Input: dimensioned drawing with shaded views. Units: mm. Origin: part minimum x, y, z. Round coordinates to 2 decimals unless told otherwise and drop trailing zeros. Loops run counter-clockwise (first coordinate to the right, second up) from the corner with the lowest first, then second, coordinate; pieces in that order, holes last.
Item 1: Section query C-C on x = 56.5. Return loops of the section in (y, z).
Item 2: Ray query, L1, parallel to X at y = 77.5, z = 1.25; L2, parallel to Y at x = 53.5, z = 5.5. Return the intervals inside material, ascending.
Item 3: Section query A-A on z = 8.5. Return loops of the section in (x, y).
Item 4: Section query B-B on y = 68.5. Return loops of the section in (x, z), then the cut area to 3 significant figures.
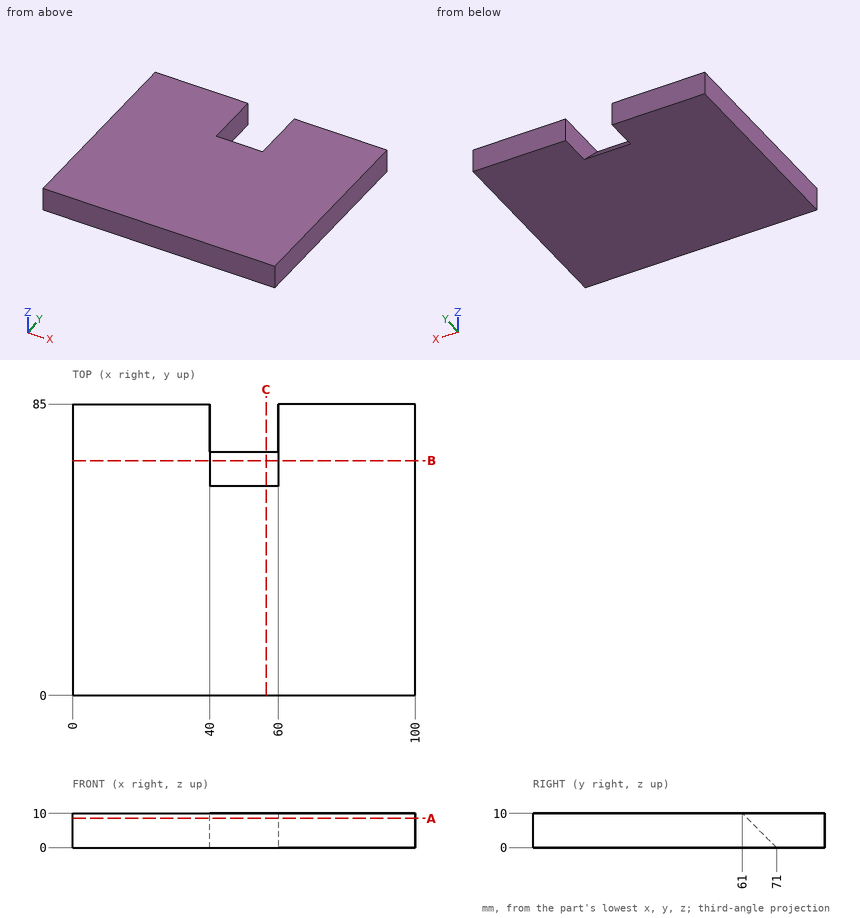
Data:
1. outline: (0, 0) - (71, 0) - (61, 10) - (0, 10) - close
2. L1: x = 0 to 40, 60 to 100
2. L2: y = 0 to 65.5
3. outline: (0, 0) - (100, 0) - (100, 85) - (60, 85) - (60, 62.5) - (40, 62.5) - (40, 85) - (0, 85) - close
4. outline: (0, 0) - (100, 0) - (100, 10) - (60, 10) - (60, 2.5) - (40, 2.5) - (40, 10) - (0, 10) - close
4. area: 850 mm2
